The listing builds one solid part. Answer for the finished solid, in the listing's coordinates (mm). A direction names the side the tool comes from. Give positions to 0.01 mm unless a question says otherwise; leave off trailing zeros. Loops run counter-clockwise (first coordinate to the right, second up) from the corner with the lowest first, then second, coordinate; pieces in that order, holes last. Notation, with made-up numbers: (-14.5, 59.5) - (35.5, 59.5) arc R29 cw to (35.5, 84.5) - close; hole circle Ø6 at (2, -34.75). An arc over 180 degrees is marked (long way). Write item = value, one per line. Start each with the question number.
1) Consider probe 1 along X at (y, z) = (-10.75, 7); probe 2 along Y at (x, z) = (5.5, -1); probe 3 along Y at (x, z) = (-14, -1.5). Determine where each line is inside the solid, lowest interval first.
2) Flat-ended cylindrical pins translate along their axes: P1, Ø2, axis at x = -16.5, y = -5, coming from the +Z side; P2, Ø5, axis at x = -22.5, z = -2, coming from the -Y side (3 decimals); P3, Ø5, axis at x = -8.5, z = -8.5, coming from the -Y side. Find the tip coordinate at first contact, or state that the pin passes through.
3) Which of the six approach directions +Z, -Z, +X, -X, +Y, -Y give full straight-line access (tool end or side, diameter ignored) to faces 1 (the flat face through (0, 7, -7)), 2 (the conical face through (8.58, 12.75, 7.56))?
4) The part is cut by section A-A on x = -7. Write down the section's boundary in (y, z) (3 decimals).
from build123d import *

# Parameters (mm, degrees)
BOSS_EXTRUDE1_DEPTH = 8.89
SKETCH2_OUTSIDE_W   = 61.52
SKETCH2_OUTSIDE_H   = 57.248
SKETCH2_OUTSIDE_R   = 14.2875
CUT_EXTRUDE1_DEPTH  = 5.08
CUT_EXTRUDE1_TAPER  = 60
SKETCH3_R           = 9.525
BOSS_EXTRUDE2_DEPTH = 31.75


with BuildPart() as part:
    # Sketch1 → Boss-Extrude1 (new body)
    with BuildSketch(Plane(origin=(0, 0, 0), x_dir=(0, 0, -1), z_dir=(1, 0, 0))):
        Polygon((8.377045531, -14.212740171), (16.497116811, 0.148364153), (8.12007128, 14.361104324), (-8.377045531, 14.212740171), (-16.497116811, -0.148364153), (-8.12007128, -14.361104324), align=None)
    extrude(amount=BOSS_EXTRUDE1_DEPTH)

    # Sketch2 outside → Cut-Extrude1 (cut)
    with BuildSketch(Plane(origin=(8.89, 0, 0), x_dir=(0, 0, -1), z_dir=(1, 0, 0))):
        Rectangle(SKETCH2_OUTSIDE_W, SKETCH2_OUTSIDE_H)
        Circle(SKETCH2_OUTSIDE_R, mode=Mode.SUBTRACT)
    extrude(amount=-CUT_EXTRUDE1_DEPTH, taper=CUT_EXTRUDE1_TAPER, mode=Mode.SUBTRACT)

    # Sketch3 → Boss-Extrude2 (add)
    with BuildSketch(Plane.ZY):
        Circle(SKETCH3_R)
    extrude(amount=BOSS_EXTRUDE2_DEPTH)


solid = part.part
Answer below:
q1.probe_1 = 0 to 8.89
q1.probe_2 = -14.28 to 14.3
q1.probe_3 = -9.41 to 9.41
q2.P1 = 8.64
q2.P2 = -9.525
q2.P3 = -7.4
q3.face_1 = -X
q3.face_2 = +Z, +X, +Y
q4.outline = circle Ø19.05 at (0, 0)
